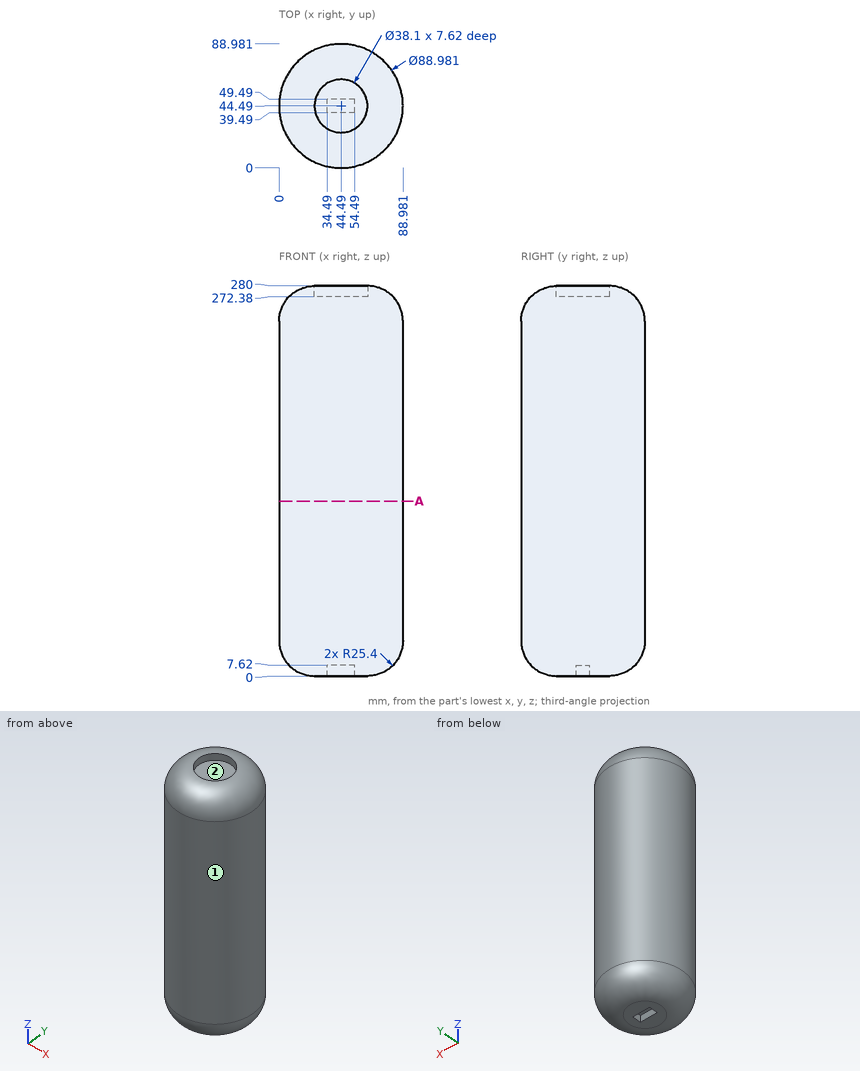
Could you check a few things on this drawing? It's one solid part, dimensions in mm from its lowest x, y, z. Give positions to 0.01 mm unless a question says otherwise; leave off trailing zeros. Order: outer loops, then holes, each group sorted by start corner. A loop starts at its lowest first (then second) coordinate and runs counter-clockwise, first axis right, second up.
1. For pin 1 (1 mm diameter, centred on y = 22, z = 153, fed in from -X) (1 decimal); pin 2 (2.5 mm diameter, centred on x = 47, z = 3, fed in from +Y) (1 decimal); pin 3 (8.5 mm diameter, centred on x = 40.5, z = 3, fed in from -Y) (1 decimal), each with a flat end and sliding along its axis, tell me the tip position at first contact or that it passes through.
Answers below:
pin 1: stops at x = 5.8
pin 2: stops at y = 77.6
pin 3: stops at y = 7.8
2. Suppose I cut it at A-A (z = 125.5). Write out the boundary of the cut face in (x, y).
Answers below:
outline: circle Ø88.98 at (44.49, 44.49)
3. Thinking about a two-plate mould opening in X: for the marked faces 1 and 2, which applies, +X half, -X half, draft (parallel to the pull), parting line (faces both ways), or undercut?
Answers below:
face 1: parting line
face 2: undercut
4. I need wall thicknesses on L1, parallel to Z at x = 39, y = 63; L2, parallel to Z at x = 45, y = 31.5; L3, parallel to X at y = 14.5, z = 64.5 (1 decimal). Which ranges of each line are inside material? Lowest first, please.
Answers below:
L1: z = 0 to 280
L2: z = 0 to 272.38
L3: x = 11.6 to 77.4
